Could you check a few things on this drawing? It's one solid part, dimensions in mm from its lowest x, y, z. Give positions to 0.01 mm unless a question says otherwise; leave off trailing zeros. Loops run counter-clockwise (first coordinate to the right, second up) from the corner with the lowest first, then second, coordinate; pieces in that order, holes last. Notation, with made-up numbers: (-1.5, 88) - (41.5, 88) arc R33 cw to (41.5, 116) - close; hole circle Ø9 at (-25.75, -27). An arc over 180 degrees is marked (long way). Write each question's results on one line, items separated by ' | '. Start each with the question number.
(1) I need wall thicknesses on line 1 (Z direction, x = 76.2, y = 2.25); line 2 (Z direction, x = 180, y = 3); line 3 (X direction, y = 2, z = 109). Which ranges of each line are inside material? Lowest first, please.
(2) Suppose I cut it at D-D (x = 159.5). Please give me the cut outline in (y, z).
(3) Suppose I cut it at A-A (x = 76.2). Please give me the cut outline in (y, z).
(4) Suppose I cut it at B-B (y = 2.5). Please give me the cut outline in (x, z).
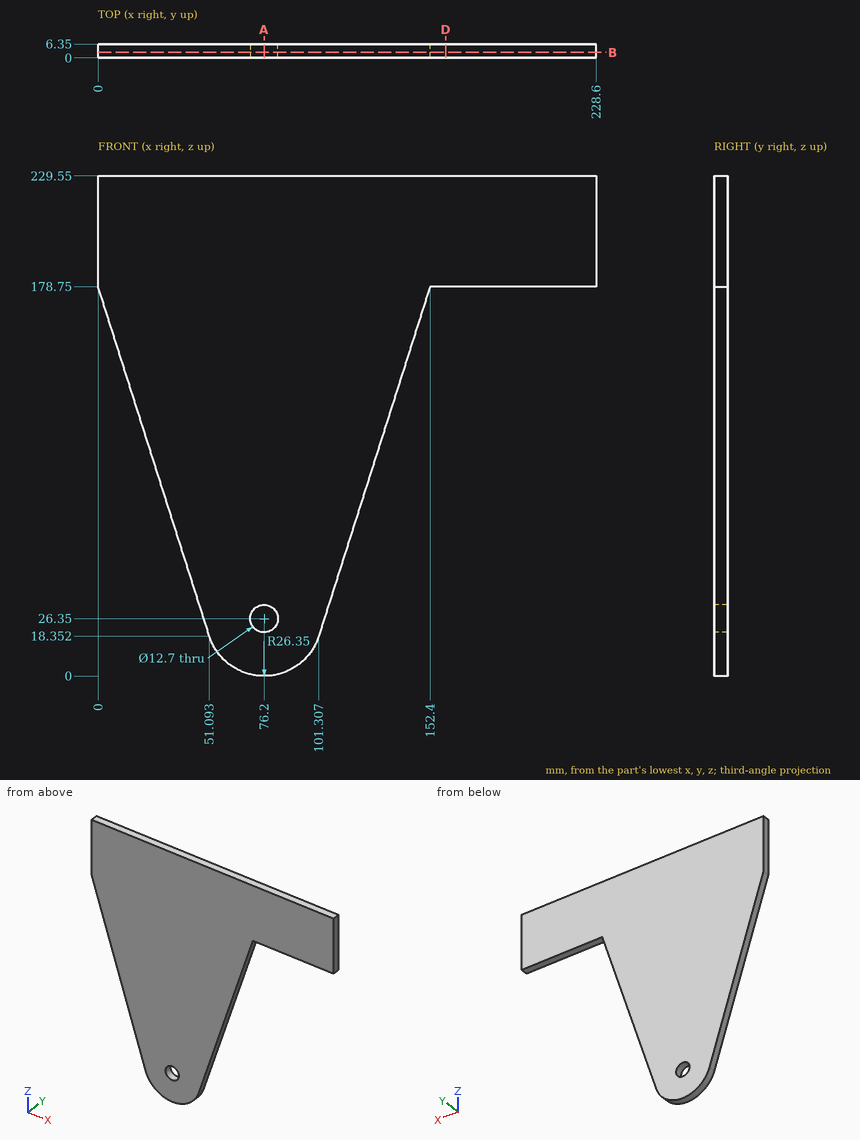
Output values:
1) line 1: 0 to 20, 32.7 to 229.55 | line 2: 178.75 to 229.55 | line 3: 22.22 to 130.18
2) outline: (0, 178.75) - (6.35, 178.75) - (6.35, 229.55) - (0, 229.55) - close
3) outline: (0, 0) - (6.35, 0) - (6.35, 20) - (0, 20) - close; (0, 32.7) - (6.35, 32.7) - (6.35, 229.55) - (0, 229.55) - close
4) outline: (0, 178.75) - (51.09, 18.35) arc R26.35 ccw to (101.31, 18.35) - (152.4, 178.75) - (228.6, 178.75) - (228.6, 229.55) - (0, 229.55) - close; hole circle Ø12.7 at (76.2, 26.35)
